Autodesk Inventor part; units mm, degrees
ref_plane "YZ Plane" through (0, 0, 0) normal (1, 0, 0) x (0, 1, 0)
ref_plane "XZ Plane" through (0, 0, 0) normal (0, 1, 0) x (-1, 0, 0)
ref_plane "XY Plane" through (0, 0, 0) normal (0, 0, 1) x (1, 0, 0)
sketch "Sketch1" plane through (0, 0, 0) normal (1, 0, 0) x (0, 1, 0)
  line L0 (0, 0) -> (101.6, 0)
  line L1 (101.6, 0) -> (101.6, -444.5)
  line L2 (101.6, -444.5) -> (0, -444.5)
  line L3 (0, -444.5) -> (0, 0)
  circle A0 centre (31.75, -50.8) radius 6.3627
  circle A1 centre (31.75, -393.7) radius 6.3627
  circle A2 centre (86.2838, -165.5318) radius 1.5875
  circle A3 centre (70.2818, -165.5318) radius 1.5875
  circle A4 centre (15.3162, -278.9682) radius 1.5875
  circle A5 centre (31.3182, -278.9682) radius 1.5875
  dimension "d0" = 101.6
  dimension "d1" = 444.5
  dimension "d2" = 12.7254
  dimension "d3" = 31.75
  dimension "d4" = 50.8
  dimension "d5" = 50.8
  dimension "d22" = 165.5318
  dimension "d23" = 3.175
  dimension "d24" = 15.3162
  dimension "d25" = 3.175
  dimension "d26" = 16.002
  dimension "d27" = 165.5318
  dimension "d28" = 3.175
  dimension "d29" = 15.3162
  dimension "d30" = 165.5318
  dimension "d31" = 3.175
  dimension "d32" = 16.002
  dimension "d33" = 165.5318
extrude "Extrusion1" add sketch "Sketch1" along normal blind 4.7625 contours L0 L1 L2 L3 | A2 | A3 | A4 | A5
chamfer "Chamfer1" distance 38.1 angle 45 1 edges at (2.3813, 0, 0)
chamfer "Chamfer2" distance 38.1 angle 45 1 edges at (2.3813, 0, -444.5)
sketch "Sketch6" plane through (4.7625, 0, 0) normal (1, 0, 0) x (0, 0, -1)
  line L0 (444.5, 38.1) -> (406.4, 0)
  line L1 (444.5, 38.1) -> (444.5, 101.6)
  line L2 (444.5, 101.6) -> (0, 101.6)
  line L3 (0, 101.6) -> (0, 38.1)
  line L4 (38.1, 0) -> (0, 38.1)
  line L5 (38.1, 0) -> (406.4, 0)
  circle A0 centre (393.7, 31.75) radius 6.3627
  circle A1 centre (50.8, 31.75) radius 6.3627
  point P0 (0, 0)
  point P1 (165.7604, 48.006)
  point P2 (165.7604, 16.002)
  point P3 (278.7396, 85.598)
  point P4 (278.7396, 53.594)
  dimension "d80" = 32.004
  dimension "d83" = 16.002
  dimension "d86" = 32.004
  dimension "d87" = 16.002
hole "Hole1" at (4.7625, 48.006, -165.7604) at (4.7625, 16.002, -165.7604) at (4.7625, 85.598, -278.7396) at (4.7625, 53.594, -278.7396) direction (-1, 0, 0) diameter 3.81 end through all
sketch "Sketch7" plane through (4.7625, 0, 0) normal (1, 0, 0) x (0, 0, -1)
  circle A0 centre (278.7396, 85.598) radius 1.905
  circle A1 centre (165.7604, 48.006) radius 1.905
  circle A2 centre (165.7604, 16.002) radius 1.905
  circle A3 centre (278.7396, 53.594) radius 1.905
  line L0 (444.5, 38.1) -> (406.4, 0)
  line L1 (444.5, 38.1) -> (444.5, 101.6)
  line L2 (444.5, 101.6) -> (0, 101.6)
  line L3 (0, 101.6) -> (0, 38.1)
  line L4 (38.1, 0) -> (0, 38.1)
  line L5 (38.1, 0) -> (406.4, 0)
  circle A4 centre (393.7, 31.75) radius 6.3627
  circle A5 centre (50.8, 31.75) radius 6.3627
  point P0 (0, 0)
  point P1 (101.6, 97.155)
  point P2 (342.9, 97.155)
  point P3 (127, 4.445)
  point P4 (317.5, 4.445)
  dimension "d95" = 4.445
  dimension "d96" = 4.445
  dimension "d97" = 4.445
  dimension "d98" = 4.445
  dimension "d99" = 101.6
  dimension "d100" = 101.6
  dimension "d101" = 127
  dimension "d102" = 127
hole "Hole2" at (4.7625, 97.155, -101.6) at (4.7625, 97.155, -342.9) at (4.7625, 4.445, -127) at (4.7625, 4.445, -317.5) direction (-1, 0, 0) diameter 3.81 depth 25.4 tip angle 118
properties part number "DriveTrain3.0" material "Aluminum 6061"
Design review of the part built by this model. Coordinates are the model's own, in mm. Coordinates: 2 decimals unless noted, no trailing zeros. Order: outer loops, then holes, each group sorted by start corner. A loop starts at its lowest first (then second) coordinate and runs counter-clockwise, first axis right, second up. Notation, with made-up numbers: (68.25, 39) -> (97.25, 39) arc R25 ccw to (97.25, 77) -> close; hole circle Ø3 at (-16, 16.5). An arc over 180 degrees is marked (long way). Use one line per item in the form item = value. Start each with the question number.
(1) Add section B-B on x = 2.75. Give the number of separate pieces and of enclosed holes in the cut face, plus the area to 3 significant figures.
(2) For probe 1 along Y at (x, z) = (1, -393.7); probe 2 along Z at (x, y) = (1.15, 31.75); probe 3 along Y at (x, z) = (2.2, -317.5), list the stretches that pass through material, from the lowest coordinate up.
(3) The part is to be moulded in two halves that separate along Z. For faces 1 (the cylindrical face through (2.35, 30.37, -44.59)), 2 (the flat face through (2.4, 19.3, -425.7)), 3 (the flat face through (4.762, 50, -219)), say which applies: +Z half, -Z half, draft (parallel to the pull), parting line (faces both ways), or undercut.
(4) Insertion check: pin 1 (4.5 mm diameter, centred on y = 85.6, z = -278.74, fed in from +X); pin 2 (1 mm diameter, centred on x = 3.5, y = 17, fed in from +Z). Each pin has a flat end and moves straight along its axis. Give the tip position at first contact, or say it passes through.
(5) Add section A-A on z = -50.8. State the section outline as (x, y) points, plus the area to 3 significant figures.
Answer block:
q1.separate_pieces = 1
q1.enclosed_holes = 10
q1.area = 43,400 mm²
q2.probe_1 = 0 to 25.39, 38.11 to 101.6
q2.probe_2 = -438.15 to -400.06, -387.34 to -57.16, -44.44 to -6.35
q2.probe_3 = 0 to 2.54, 6.35 to 101.6
q3.face_1 = undercut
q3.face_2 = -Z half
q3.face_3 = draft
q4.pin_1 = 4.76
q4.pin_2 = -20.6
q5.outline = (0, 0) -> (4.76, 0) -> (4.76, 25.39) -> (0, 25.39) -> close; (0, 38.11) -> (4.76, 38.11) -> (4.76, 101.6) -> (0, 101.6) -> close
q5.area = 423 mm²
